from build123d import *

# Parameters (mm, degrees)
PAD_DEPTH            = 56
PAD001_DEPTH         = 56
FILLET_R             = 4.5
SKETCH001_R          = 7.9375
SKETCH001_R_2        = 2
POCKET_DEPTH         = 50.801
LINEARPATTERN_COUNT  = 2
LINEARPATTERN_PITCH  = 80
SKETCH002_R          = 5.357812
SKETCH002_R_2        = 1.5875
POCKET001_DEPTH      = 50.801
POCKET001_DEPTH_BACK = 0.001
SKETCH003_W          = 60
SKETCH003_H          = 51.1187
POCKET002_DEPTH      = 266.123378
POCKET002_DEPTH_BACK = 316.923378
SKETCH004_R          = 1.865
SKETCH004_R_2        = 11.1125
POCKET003_DEPTH      = 0.001
POCKET003_DEPTH_BACK = 50.801
SKETCH005_W          = 60
SKETCH005_H          = 12.25
POCKET004_DEPTH      = 56.001
POCKET004_DEPTH_BACK = 56.001
SKETCH006_W          = 37.3666
SKETCH006_H          = 44.7638
POCKET005_DEPTH      = 266.123378
POCKET005_DEPTH_BACK = 316.923378


with BuildPart() as part:
    # Sketch → Pad (new body)
    with BuildSketch(Plane.XY):
        Polygon((0, 0), (50.8, 0), (50.8, -6.35), (6.35, -6.35), (6.35, -50.8), (0, -50.8), align=None)
    extrude(amount=-PAD_DEPTH)

    # Sketch → Pad001 (join)
    with BuildSketch(Plane.XY):
        Polygon((0, 0), (50.8, 0), (50.8, -6.35), (6.35, -6.35), (6.35, -50.8), (0, -50.8), align=None)
    extrude(amount=PAD001_DEPTH)

    # Fillet
    fillet_edges = [part.edges().sort_by_distance(p)[0] for p in [
        (6.35, -50.8, 0),
        (6.35, -6.35, 0),
        (50.8, -6.35, 0),
    ]]
    fillet(fillet_edges, radius=FILLET_R)

    # Sketch001 → Pocket (cut, through all)
    with BuildSketch(Plane.YZ):
        with Locations((-14, -40)):
            Circle(SKETCH001_R)
        with Locations((-14, -28)):
            Circle(SKETCH001_R_2)
        with Locations((-14, -52)):
            Circle(SKETCH001_R_2)
    pocket = extrude(amount=POCKET_DEPTH, mode=Mode.SUBTRACT)

    # LinearPattern: Pocket ×2
    with Locations(*[(0, 0, i * LINEARPATTERN_PITCH) for i in range(1, LINEARPATTERN_COUNT)]):
        add(pocket, mode=Mode.SUBTRACT)

    # Sketch002 → Pocket001 (cut, two sides)
    with BuildSketch(Plane.YZ) as pocket001_sk:
        with Locations((-39, 0)):
            Circle(SKETCH002_R)
        with Locations((-44.656854, 5.656854)):
            Circle(SKETCH002_R_2)
        with Locations((-33.343146, 5.656854)):
            Circle(SKETCH002_R_2)
        with Locations((-33.343146, -5.656854)):
            Circle(SKETCH002_R_2)
        with Locations((-44.656854, -5.656854)):
            Circle(SKETCH002_R_2)
    extrude(amount=POCKET001_DEPTH, mode=Mode.SUBTRACT)
    extrude(pocket001_sk.sketch, amount=-POCKET001_DEPTH_BACK, mode=Mode.SUBTRACT)

    # Sketch003 → Pocket002 (cut, two sides)
    with BuildSketch(Plane.XZ) as pocket002_sk:
        with Locations((36.35, 50.55935)):
            Rectangle(SKETCH003_W, SKETCH003_H)
    pocket002 = extrude(amount=-POCKET002_DEPTH, mode=Mode.SUBTRACT) + extrude(pocket002_sk.sketch, amount=POCKET002_DEPTH_BACK, mode=Mode.SUBTRACT)

    # Mirrored001: Pocket002 across Sketch003 H_Axis
    add(pocket002.mirror(Plane(origin=(0, 0, 0), x_dir=(0, -1, 0), z_dir=(0, 0, 1))), mode=Mode.SUBTRACT)

    # Sketch004 → Pocket003 (cut, two sides)
    with BuildSketch(Plane.XZ) as pocket003_sk:
        with Locations((43.5, 15.5)):
            Circle(SKETCH004_R)
        with Locations((43.5, -15.5)):
            Circle(SKETCH004_R)
        with Locations((12.5, 15.5)):
            Circle(SKETCH004_R)
        with Locations((12.5, -15.5)):
            Circle(SKETCH004_R)
        with Locations((28, 0)):
            Circle(SKETCH004_R_2)
    extrude(amount=-POCKET003_DEPTH, mode=Mode.SUBTRACT)
    extrude(pocket003_sk.sketch, amount=POCKET003_DEPTH_BACK, mode=Mode.SUBTRACT)

    # Sketch005 → Pocket004 (cut, two sides)
    with BuildSketch(Plane.XY) as pocket004_sk:
        with Locations((36.35, -10.8875)):
            Rectangle(SKETCH005_W, SKETCH005_H)
    extrude(amount=-POCKET004_DEPTH, mode=Mode.SUBTRACT)
    extrude(pocket004_sk.sketch, amount=POCKET004_DEPTH_BACK, mode=Mode.SUBTRACT)

    # Sketch006 → Pocket005 (cut, two sides)
    with BuildSketch(Plane.YZ) as pocket005_sk:
        with Locations((-43.4833, 47.3819)):
            Rectangle(SKETCH006_W, SKETCH006_H)
    pocket005 = extrude(amount=-POCKET005_DEPTH, mode=Mode.SUBTRACT) + extrude(pocket005_sk.sketch, amount=POCKET005_DEPTH_BACK, mode=Mode.SUBTRACT)

    # Mirrored: Pocket005 across Sketch006 H_Axis
    add(pocket005.mirror(Plane.XY), mode=Mode.SUBTRACT)


solid = part.part
Read the model definition and answer for the solid it produces. Units are mm, in the model's axes. A direction names the side the tool comes from. Round coordinates to 2 decimals unless told otherwise and drop trailing zeros. Loops run counter-clockwise (first coordinate to the right, second up) from the corner with the lowest first, then second, coordinate; pieces in that order, holes last.
Q1. Which of the six approach directions +Z, -Z, +X, -X, +Y, -Y give full straight-line access (tool end or side, diameter ignored) to faces 1 (the face through (3, -38, 25)), 2 (the face through (28, -2, -25)), 3 (the face through (3, -24.8, -40)), 4 (the face through (3, -12, 56))?
Q2. Section D-D on z = -15.5 is taken. Give the number of separate pieces and of enclosed holes in the cut face, and give its area (3 significant figures).
Q3. Determine the mould class of faces 5 (the face through (6.35, -18, -1)), 6 (the face through (27.7, -4.762, 11.5)), 7 (the face through (3.131, -13.077, 26.226)) for opening direction Y: released by +Y, released by -Y, zero draft, split by the parting line, or undercut.
Q4. Section C-C on y = -39 is taken. Write down the section's boundary in (x, z), and give its area (3 significant figures).
Q5. Section A-A on z = 28 is taken. Write down the section's boundary in (x, y).
Q6. Section B-B on x = 43.5 is taken. Write down the section's boundary in (y, z) (1 decimal), and give its area (3 significant figures).
Q7. Consider probe 1 along Z at (x, y) = (12.5, -3.75) (3 decimals); probe 2 along Y at (x, z) = (2, -40); probe 3 along Y at (x, z) = (4.75, -28). Determine where each line is inside the solid, lowest interval first.
Q8. Each of these flat-tipped pins is pushed along its axis until it touches: pin 1 (6 mm diameter, centred on y = -17, z = -26, fed in from +X); pin 2 (7 mm diameter, centred on x = 4, y = -35, fed in from -Z); pin 3 (7 mm diameter, centred on x = 2.5, y = -41.5, fed in from +Z). Where does it stop, or does it pass through?
Output:
1. face 1: +Z, +X, -X, -Y
1. face 2: -Z, +X, +Y, -Y
1. face 3: -Z, +X, -X, -Y
1. face 4: +Z, +X, -X, +Y, -Y
2. separate pieces: 3
2. enclosed holes: 0
2. area: 493 mm2
3. face 5: zero draft
3. face 6: released by -Y
3. face 7: undercut
4. outline: (0, -25) - (6.35, -25) - (6.35, -5.36) - (0, -5.36) - close; (0, 5.36) - (6.35, 5.36) - (6.35, 25) - (0, 25) - close
4. area: 249 mm2
5. outline: (0, -24.8) - (6.35, -24.8) - (6.35, -16) - (0, -16) - close; (0, -12) - (6.35, -12) - (6.35, 0) - (0, 0) - close
6. outline: (-4.8, -25) - (0, -25) - (0, -17.4) - (-4.8, -17.4) - close; (-4.8, -13.6) - (0, -13.6) - (0, 13.6) - (-4.8, 13.6) - close; (-4.8, 17.4) - (0, 17.4) - (0, 25) - (-4.8, 25) - close
6. area: 203 mm2
7. probe 1: z = -25 to -17.365, -13.635 to 13.635, 17.365 to 25
7. probe 2: y = -24.8 to -21.94, -6.06 to 0
7. probe 3: y = -24.8 to -16, -12 to 0
8. pin 1: stops at x = 6.35
8. pin 2: stops at z = -25
8. pin 3: stops at z = 25
